For this review, take the finished solid that the model builds, in its own axes (mm). A direction names the side the tool comes from. Give positions to 0.01 mm unless a question says otherwise; leave off trailing zeros. Write each loop counter-clockwise with the first axis right and the second up, starting at its lowest first coordinate (ties: lowest second). Pieces come first, ordered by that corner, then holes.
1) We need section A-A on z = 7.5. Give the boundary of the cut face in (x, y).
2) Machinability: for faces 5 (the face through (-6.65, -7, 6)), 6 (the face through (-1, -8, 7)), 7 (the face through (0.19, 8.648, 7.395)), 8 (the face through (7, -2.726, 7)), 9 (the face through (3.36, -5.18, 6.17)), which of the approach directions +Z, -Z, +X, -X, +Y, -Y give a long, thin tool a straight path to every point of the face, cutting with its end or side? Answer none if there is none.
3) Draft analysis for pull direction Y (two halves, no side actions). For faces 1 (the face through (5, -11.751, 7)), 2 (the face through (-8.65, -3, 9)), 3 (the face through (7, -9.026, 8)), 4 (the face through (7.17, -7.43, 10.24)), state which applies: pulls with the +Y half, pulls with the -Y half, needs draft (parallel to the pull), parting line crosses it, or undercut.
4) Wall thickness on line 1 along X through (y, z) = (-7.75, 6.25); line 2 along X through (y, z) = (-7, 14.25); line 3 along Y through (x, z) = (-2.5, 12.5): over which ranges is each line inside the solid? List them lowest first.
5) We need section C-C on y = -6.75. Give the boundary of the cut face in (x, z).
6) For P1, Ø6, axis at y = -5, z = 8.5, coming from the -X side; P2, Ø3.5, axis at y = -5.88, z = 7.5, coming from the +X side; P3, Ø4.5, axis at y = -5.88, z = 7.5, coming from the -X side; P4, Ø1, axis at x = -5.5, z = 5.5, coming from the +Y side, all flat-tipped, find the tip position at first contact; note any pin that passes through.
7) We need section D-D on y = 1. Give the boundary of the cut face in (x, z), and give its area (3 significant figures).
8) We need section B-B on x = 2.25. Give the boundary of the cut face in (y, z).
from build123d import *

# Parameters (mm, degrees)
F1_DEPTH = 15
F2_R     = 1.5
F3_DEPTH = 17.301
F5_DEPTH = 3
F6_R     = 2.75
F7_DEPTH = 2


with BuildPart() as f1:
    # F0 (on Top) → F1 (new body)
    with BuildSketch(Plane.XY):
        with BuildLine():
            Line((-1, -11.7513947189), (-1, -8.592002095))
            ThreePointArc((-1, -8.592002095), (-6.4603598971, -5.7520648466), (-8.65, 0))
            Line((-8.65, 0), (-8.65, -11.7513947189))
            Line((-8.65, -11.7513947189), (-1, -11.7513947189))
        make_face()
        with BuildLine():
            ThreePointArc((8.65, 0), (6.4603598971, -5.7520648466), (1, -8.592002095))
            Line((1, -8.592002095), (1, -11.7513947189))
            Line((1, -11.7513947189), (8.65, -11.7513947189))
            Line((8.65, -11.7513947189), (8.65, 0))
        make_face()
        with BuildLine():
            Line((-8.65, 0), (-4.15, 0))
            ThreePointArc((-4.15, 0), (0, 4.15), (4.15, 0))
            Line((4.15, 0), (8.65, 0))
            ThreePointArc((8.65, 0), (0, 8.65), (-8.65, 0))
        make_face()
        with BuildLine():
            Line((-1, -8.592002095), (-1, -4.0277164746))
            ThreePointArc((-1, -4.0277164746), (-3.2689830223, -2.5566090824), (-4.15, 0))
            Line((-4.15, 0), (-8.65, 0))
            ThreePointArc((-8.65, 0), (-6.4603598971, -5.7520648466), (-1, -8.592002095))
        make_face()
        with BuildLine():
            ThreePointArc((4.15, 0), (3.2689830223, -2.5566090824), (1, -4.0277164746))
            Line((1, -4.0277164746), (1, -8.592002095))
            ThreePointArc((1, -8.592002095), (6.4603598971, -5.7520648466), (8.65, 0))
            Line((8.65, 0), (4.15, 0))
        make_face()
    extrude(amount=F1_DEPTH)

    # F2 (on face) → F3 (cut, through all)
    with BuildSketch(Plane.YZ.offset(8.65)):
        with Locations((-5.8756973594, 7.5)):
            Circle(F2_R)
    extrude(amount=-F3_DEPTH, mode=Mode.SUBTRACT)

    # F4 (on face) → F5 (cut)
    with BuildSketch(Plane.YZ.offset(8.65)):
        Polygon((-2.7256973594, 9.3186533479), (-5.8756973594, 11.1373066959), (-9.0256973594, 9.3186533479), (-9.0256973594, 5.6813466521), (-5.8756973594, 3.8626933041), (-2.7256973594, 5.6813466521), align=None)
    extrude(amount=-F5_DEPTH, mode=Mode.SUBTRACT)

    # F6 (on face) → F7 (cut)
    with BuildSketch(Plane(origin=(-8.65, 0, 0), x_dir=(0, -1, 0), z_dir=(-1, 0, 0))):
        with Locations((5.8756973594, 7.5)):
            Circle(F6_R)
    extrude(amount=-F7_DEPTH, mode=Mode.SUBTRACT)


solid = f1.part
Results list:
1. outline: (-8.65, -11.75) - (-1, -11.75) - (-1, -7.38) - (-6.65, -7.38) - (-6.65, -8.63) - (-8.65, -8.63) - close; (-8.65, -3.13) - (-6.65, -3.13) - (-6.65, -4.38) - (-1, -4.38) - (-1, -4.03) arc R4.15 cw (long way) to (1, -4.03) - (1, -4.38) - (5.65, -4.38) - (5.65, -2.73) - (8.65, -2.73) - (8.65, 0) arc R8.65 ccw to (-8.65, 0) - close; (1, -11.75) - (8.65, -11.75) - (8.65, -9.03) - (5.65, -9.03) - (5.65, -7.38) - (1, -7.38) - close
2. face 5: -X
2. face 6: +Z, -Z, -Y
2. face 7: +Z, -Z, +Y
2. face 8: +X
2. face 9: +X, -X
3. face 1: pulls with the -Y half
3. face 2: needs draft
3. face 3: undercut
3. face 4: undercut
4. line 1: x = -6.65 to -1, 1 to 5.65
4. line 2: x = -8.65 to -1, 1 to 8.65
4. line 3: y = -11.75 to -3.31, 3.31 to 8.28
5. outline: (-8.65, 0) - (-1, 0) - (-1, 6.28) - (-6.65, 6.28) - (-6.65, 4.89) - (-8.65, 4.89) - close; (-8.65, 10.11) - (-6.65, 10.11) - (-6.65, 8.72) - (-1, 8.72) - (-1, 15) - (-8.65, 15) - close; (1, 0) - (8.65, 0) - (8.65, 4.37) - (5.65, 4.37) - (5.65, 6.28) - (1, 6.28) - close; (1, 8.72) - (5.65, 8.72) - (5.65, 10.63) - (8.65, 10.63) - (8.65, 15) - (1, 15) - close
6. P1: stops at x = -8.65
6. P2: stops at x = 5.65
6. P3: stops at x = -6.65
6. P4: stops at y = 7.06
7. outline: (-8.59, 0) - (-4.03, 0) - (-4.03, 15) - (-8.59, 15) - close; (4.03, 0) - (8.59, 0) - (8.59, 15) - (4.03, 15) - close
7. area: 137 mm2
8. outline: (-11.75, 0) - (-3.49, 0) - (-3.49, 15) - (-11.75, 15) - close; (3.49, 0) - (8.35, 0) - (8.35, 15) - (3.49, 15) - close; hole circle Ø3 at (-5.88, 7.5)
